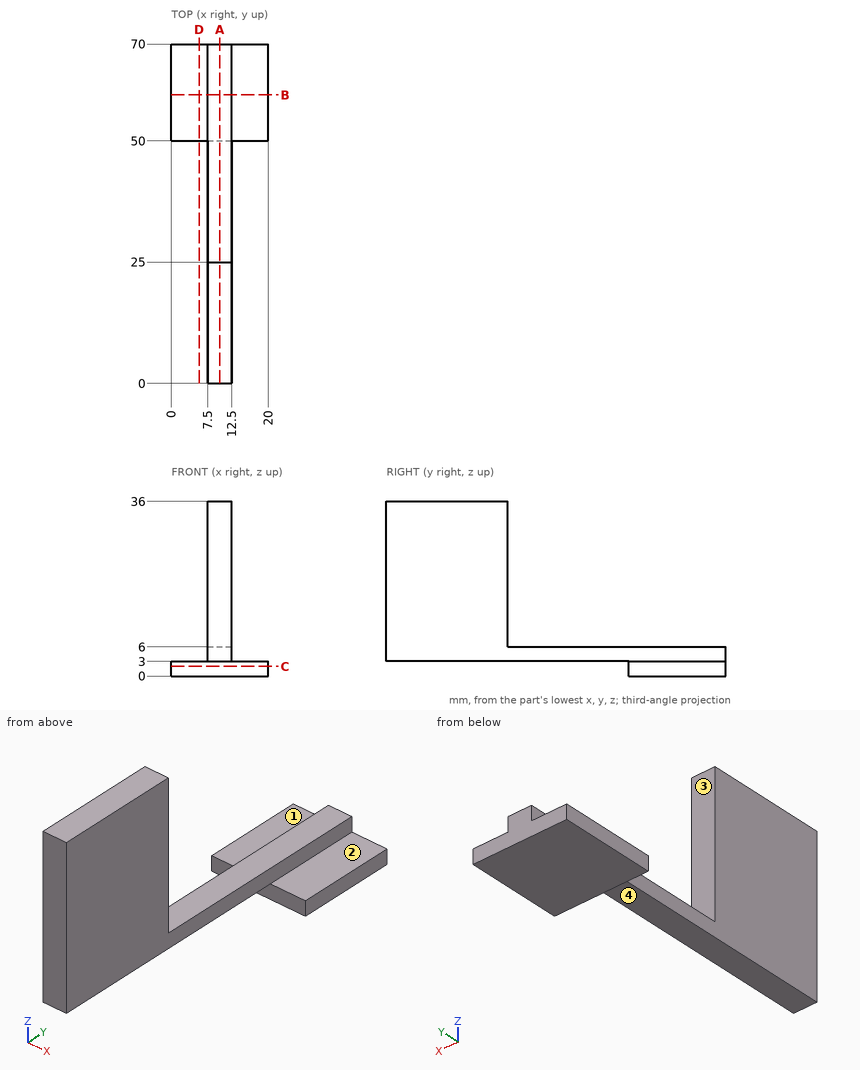
Can you work these out from the drawing? Everything is in mm from the part's minimum corner. A direction names the side the tool comes from. Round coordinates to 2 decimals unless told otherwise and drop trailing zeros. Loops run counter-clockwise (first coordinate to the right, second up) from the corner with the lowest first, then second, coordinate; pieces in that order, holes last. Notation, with made-up numbers: (-2, 83) - (11, 83) arc R14 cw to (11, 109) - close; hole circle Ø9 at (0.5, -3.5). An arc over 180 degrees is marked (long way). Answer in a Markdown table with one row per item. Add a question column.
Q1. I want a section at C-C on z = 2. List the corners of the cut face in (x, y) for me, and give its area (3 significant figures).
Q2. I want a section at A-A on x = 10. List the corners of the cut face in (y, z) for me, and give its area (3 significant figures).
Q3. I want a section at B-B on y = 59.5. List the corners of the cut face in (x, z) for me.
Q4. I need wall thicknesses on L1, parallel to Z at x = 1, y = 61; L2, parallel to X at y = 21.5, z = 17.5; L3, parallel to Z at x = 8.5, y = 64. Which ranges of each line are inside material? Lowest first, please.
Q5. I want a section at D-D on x = 5.75. List the corners of the cut face in (y, z) for me, and give its area (3 significant figures).
Q6. For pin 1 Ø4 at (x, z) = (9.5, 19.5) entering from +Y; pin 2 Ø6 at (x, y) = (14.5, 58.5) entering from +Z; pin 3 Ø0.9 at (x, z) = (12.5, 1.5) entering from -Y; pin 4 Ø6 at (y, z) = (60, 5) entering from +X, each with a flat end and sliding along its axis, tell me the tip position at first contact or that it passes through.
Q7. Which directions (+Z, -Z, +X, -X, +Y, -Y) give clear straight access to the entire face, cutting with the end or side of a thin tool? Please do the marked faces 1, 2, 3 and 4.
A:
| question | item | result |
|---|---|---|
| 1 | outline | (0, 50) - (20, 50) - (20, 70) - (0, 70) - close |
| 1 | area | 400 mm^2 |
| 2 | outline | (0, 3) - (50, 3) - (50, 0) - (70, 0) - (70, 6) - (25, 6) - (25, 36) - (0, 36) - close |
| 2 | area | 1,020 mm^2 |
| 3 | outline | (0, 0) - (20, 0) - (20, 3) - (12.5, 3) - (12.5, 6) - (7.5, 6) - (7.5, 3) - (0, 3) - close |
| 4 | L1 | 0 to 3 |
| 4 | L2 | 7.5 to 12.5 |
| 4 | L3 | 0 to 6 |
| 5 | outline | (50, 0) - (70, 0) - (70, 3) - (50, 3) - close |
| 5 | area | 60.0 mm^2 |
| 6 | pin 1 | y = 25 |
| 6 | pin 2 | z = 6 |
| 6 | pin 3 | y = 50 |
| 6 | pin 4 | x = 20 |
| 7 | face 1 | +Z, -X, +Y, -Y |
| 7 | face 2 | +Z, +X, +Y, -Y |
| 7 | face 3 | +Z, +X, -X, +Y |
| 7 | face 4 | -Z, +X, -X, -Y |
